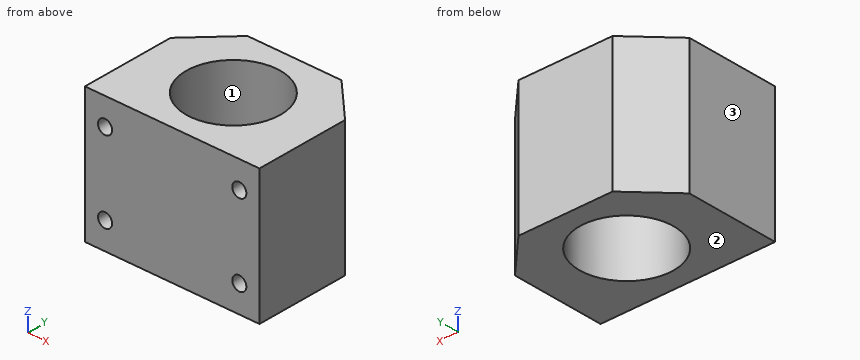
from build123d import *

# Parameters (mm, degrees)
SKETCH1_R           = 14
BOSS_EXTRUDE1_DEPTH = 40
SKETCH2_R           = 2.1
CUT_EXTRUDE1_DEPTH  = 10


with BuildPart() as part:
    # Sketch1 → Boss-Extrude1 (new body)
    with BuildSketch(Plane.XY):
        Polygon((-14, 20), (14, 20), (26, 8), (26, -20), (-26, -20), (-26, 8), align=None)
        Circle(SKETCH1_R, mode=Mode.SUBTRACT)
    extrude(amount=BOSS_EXTRUDE1_DEPTH)

    # Sketch2 → Cut-Extrude1 (cut)
    with BuildSketch(Plane.XZ.offset(20)):
        with Locations((-20, 32)):
            Circle(SKETCH2_R)
        with Locations((20, 32)):
            Circle(SKETCH2_R)
        with Locations((20, 8)):
            Circle(SKETCH2_R)
        with Locations((-20, 8)):
            Circle(SKETCH2_R)
    extrude(amount=-CUT_EXTRUDE1_DEPTH, mode=Mode.SUBTRACT)


solid = part.part
Could you check a few things on this model? Use its own coordinates, in mm. Face numbers are marked on the shaded views. Give positions to 0.01 mm unless a question says otherwise; leave off trailing zeros. Write each loop counter-clockwise with the first axis right and the second up, starting at its lowest first coordinate (ties: lowest second). Pieces come first, ordered by that corner, then holes. Notation, with made-up numbers: (42.5, 43) -> (67.5, 43) arc R17 cw to (67.5, 53) -> close; hole circle Ø9 at (-21, 47). An arc over 180 degrees is marked (long way). Answer as CSV lines item,"result". Start each with the question number.
(1) If we section it at A-A, the plane z = 32: Write out the boundary of the cut face in (x, y), and give its area (3 significant figures).
(2) If we mould it in two halves opening along X, with no side actions, what happens to the marked faces 1, 2 and 3? For each: +X half, -X half, draft (parallel to the pull), parting line (faces both ways), or undercut.
(3) If we section it at D-D, the plane y = -11.5: Write out the boundary of the cut face in (x, z).
(4) If we section it at C-C, the plane y = -2: Write out the boundary of the cut face in (x, z).
(5) Please list where these lines run through material, in increasing order: line 1 (Z direction, x = 20, y = -14); line 2 (Z direction, x = 21.5, y = -14.5); line 3 (Y direction, x = -1.5, z = 19.5).
(6) I'm going to push flat-ended pins straight in: pin 1 Ø5 at (x, z) = (20, 32) entering from +Y; pin 2 Ø2 at (x, z) = (-20.5, 32.5) entering from -Y. Where does each tip first touch, or does it pass through?
(7) If we section it at B-B, the plane x = 0: Write out the boundary of the cut face in (y, z), and give its area (3 significant figures).
Answer list:
1,outline,"(-26, -20) -> (-22.1, -20) -> (-22.1, -10) -> (-17.9, -10) -> (-17.9, -20) -> (17.9, -20) -> (17.9, -10) -> (22.1, -10) -> (22.1, -20) -> (26, -20) -> (26, 8) -> (14, 20) -> (-14, 20) -> (-26, 8) -> close; hole circle Ø28 at (0, 0)"
1,area,"1,240 mm^2"
2,face 1,"undercut"
2,face 2,"draft"
2,face 3,"-X half"
3,outline,"(-26, 0) -> (-7.98, 0) -> (-7.98, 40) -> (-26, 40) -> close; (7.98, 0) -> (26, 0) -> (26, 40) -> (7.98, 40) -> close; hole circle Ø4.2 at (-20, 8); hole circle Ø4.2 at (-20, 32); hole circle Ø4.2 at (20, 8); hole circle Ø4.2 at (20, 32)"
4,outline,"(-26, 0) -> (-13.86, 0) -> (-13.86, 40) -> (-26, 40) -> close; (13.86, 0) -> (26, 0) -> (26, 40) -> (13.86, 40) -> close"
5,line 1,"0 to 5.9, 10.1 to 29.9, 34.1 to 40"
5,line 2,"0 to 6.53, 9.47 to 30.53, 33.47 to 40"
5,line 3,"-20 to -13.92, 13.92 to 20"
6,pin 1,"y = 16.5"
6,pin 2,"y = -10"
7,outline,"(-20, 0) -> (-14, 0) -> (-14, 40) -> (-20, 40) -> close; (14, 0) -> (20, 0) -> (20, 40) -> (14, 40) -> close"
7,area,"480 mm^2"
